Here's how the part is built. I have some questions about the finished solid (model axes, mm). Face numbers are marked on the shaded views. Round coordinates to 2 decimals unless told otherwise and drop trailing zeros. Write each loop counter-clockwise with the first axis right and the second up, starting at its lowest first coordinate (ties: lowest second). Pieces come first, ordered by that corner, then holes. Notation, with made-up numbers: (-25, -35.5) -> (19, -35.5) arc R19 cw to (19, -24.5) -> close; hole circle Ø8 at (-16.75, 4). An arc over 180 degrees is marked (long way). Put each result on its own line as item: value. Start each with the question number.
1. For pin 1 (1.5 mm diameter, centred on x = -34.5, z = 0.5, fed in from +Y); pin 2 (0.9 mm diameter, centred on y = -66.5, z = 1, fed in from -X); pin 3 (10.5 mm diameter, centred on x = 28.2, y = -65.37, fed in from +Z); pin 4 (1.5 mm diameter, centred on y = -73.5, z = 1, fed in from +X), each with a flat end and sliding along its axis, tell me the tip position at first contact or that it passes through.
2. Suppose I cut it at A-A (y = 0). Please give me the cut outline in (x, z).
3. I need wall thicknesses on probe 1 along X at (y, z) = (0, 1.45); probe 2 along Y at (x, z) = (23.5, 0.95); probe 3 along Y at (x, z) = (24, 1.45). Which ranges of each line are inside material? Lowest first, please. Write a range as from..to.
4. We'd pull the mould along Z, two halves only. Please class the marked faces 1 and 2: +Z half, -Z half, draft (parallel to the pull), parting line (faces both ways), or undercut.
5. Suppose I cut it at B-B (x = 29.5). Please give me the cut outline in (y, z).
6. Suppose I cut it at C-C (z = 0.5). Please give me the cut outline in (x, y).
7. Suppose I cut it at D-D (y = -36.5). Please give me the cut outline in (x, z), then the cut area to 3 significant figures.
```python
from build123d import *

# Parameters (mm, degrees)
ESQUISSE1_R        = 4
BOSS_EXTRU_1_DEPTH = 3


with BuildPart() as part:
    # Esquisse1 → Boss.-Extru.1 (new body)
    with BuildSketch(Plane.XY):
        with BuildLine():
            Line((-21.034238815, -57.791096178), (-21.034238815, -81.072422518))
            ThreePointArc((-21.034238815, -81.072422518), (-29.215924567, -78.495902105), (-37.091180109, -75.096080148))
            Line((-37.091180109, -75.096080148), (-37.091180109, -69.056201422))
            ThreePointArc((-37.091180109, -69.056201422), (-38.665509003, -62.366556039), (-43.058027489, -57.081137592))
            ThreePointArc((-43.058027489, -57.081137592), (0, 71.5), (43.058027489, -57.081137592))
            ThreePointArc((43.058027489, -57.081137592), (38.665509003, -62.366556039), (37.091180109, -69.056201422))
            Line((37.091180109, -69.056201422), (37.091180109, -75.096080148))
            ThreePointArc((37.091180109, -75.096080148), (29.215924567, -78.495902105), (21.034238815, -81.072422518))
            Line((21.034238815, -81.072422518), (21.034238815, -57.791096178))
            ThreePointArc((21.034238815, -57.791096178), (0, 61.5), (-21.034238815, -57.791096178))
        make_face()
        with Locations((-28.202703448, -65.371545378)):
            Circle(ESQUISSE1_R, mode=Mode.SUBTRACT)
        with Locations(Location((28.202703448, -65.371545378, 0), (0, 0, 180))):
            Circle(ESQUISSE1_R, mode=Mode.SUBTRACT)
    extrude(amount=BOSS_EXTRU_1_DEPTH)


solid = part.part
```
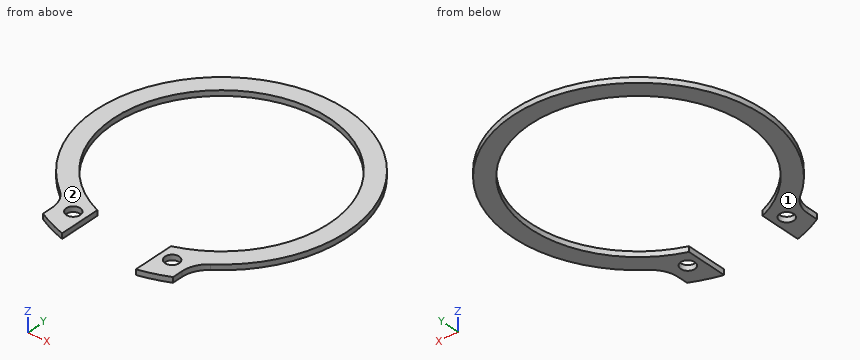
Verdict:
1. pin 1: stops at y = 63.03
1. pin 2: stops at x = -37.4
1. pin 3: stops at z = 3
1. pin 4: stops at x = 37.09
2. outline: (-71.5, 0) -> (-61.5, 0) -> (-61.5, 3) -> (-71.5, 3) -> close; (61.5, 0) -> (71.5, 0) -> (71.5, 3) -> (61.5, 3) -> close
3. probe 1: x = -71.5..-61.5, 61.5..71.5
3. probe 2: y = -80.39..-56.83, 56.83..67.53
3. probe 3: y = -80.24..-56.62, 56.62..67.35
4. face 1: -Z half
4. face 2: +Z half
5. outline: (-78.39, 0) -> (-69.16, 0) -> (-69.16, 3) -> (-78.39, 3) -> close; (-61.59, 0) -> (-53.96, 0) -> (-53.96, 3) -> (-61.59, 3) -> close; (53.96, 0) -> (65.13, 0) -> (65.13, 3) -> (53.96, 3) -> close
6. outline: (-43.06, -57.08) arc R15 cw to (-37.09, -69.06) -> (-37.09, -75.1) arc R83.76 ccw to (-21.03, -81.07) -> (-21.03, -57.79) arc R61.5 cw (long way) to (21.03, -57.79) -> (21.03, -81.07) arc R83.76 ccw to (37.09, -75.1) -> (37.09, -69.06) arc R15 cw to (43.06, -57.08) arc R71.5 ccw (long way) to start; hole circle Ø8 at (-28.2, -65.37); hole circle Ø8 at (28.2, -65.37)
7. outline: (-61.48, 0) -> (-49.5, 0) -> (-49.5, 3) -> (-61.48, 3) -> close; (49.5, 0) -> (61.48, 0) -> (61.48, 3) -> (49.5, 3) -> close
7. area: 71.9 mm^2
